Autodesk Inventor part; units mm, degrees
ref_plane "YZ Plane" through (0, 0, 0) normal (1, 0, 0) x (0, 1, 0)
ref_plane "XZ Plane" through (0, 0, 0) normal (0, 1, 0) x (-1, 0, 0)
ref_plane "XY Plane" through (0, 0, 0) normal (0, 0, 1) x (1, 0, 0)
sketch "草圖4" plane through (0, 0, 0) normal (0, 0, 1) x (1, 0, 0)
  line L0 (-29.4, 0) -> (29.4, 0)
  line L1 (0, -7) -> (0, 7)
  line L2 (-21, 5) -> (21, 5)
  line L3 (21, 5) -> (21, -5)
  line L4 (21, -5) -> (-21, -5)
  line L5 (-21, -5) -> (-21, 5)
  circle A0 centre (-11, 0) radius 1.65
  circle A1 centre (11, 0) radius 1.65
  point P0 (0, 0)
  dimension "d20" = 42
  dimension "d21" = 10
  dimension "d22" = 3.3
  dimension "d23" = 3.3
  dimension "d24" = 10
  dimension "d25" = 10
extrude "擠出3" add sketch "草圖4" along normal mid plane 23.5 contours L5 L2 L1 L0 A0 | L0 A0 L1 L4 L5 | L1 L0 A1 L3 L4 | L2 L3 L0 A1 L1
sketch "草圖5" plane through (-21, 5, 11.75) normal (0, 1, 0) x (1, 0, 0)
  line L0 (0, 0) -> (0, 23.5)
  line L1 (42, 0) -> (0, 0)
  line L2 (42, 23.5) -> (42, 0)
  line L3 (0, 23.5) -> (42, 23.5)
  circle A0 centre (21, 11.75) radius 8.5
  circle A1 centre (4.125, 19.25) radius 1.65
  circle A2 centre (4.125, 6.25) radius 1.65
  line L4 (42, 23.5) -> (0, 23.5)
  line L5 (21, 23.5) -> (21, 25.0136)
  circle A3 centre (37.875, 19.25) radius 1.65
  circle A4 centre (37.875, 6.25) radius 1.65
  circle A5 centre (4.125, 19.25) radius 3
  circle A6 centre (4.125, 6.25) radius 3
  circle A7 centre (37.875, 19.25) radius 3
  circle A8 centre (37.875, 6.25) radius 3
  dimension "d28" = 17
  dimension "d31" = 3.3
  dimension "d32" = 3.3
  dimension "d33" = 4.125
  dimension "d34" = 4.25
  dimension "d35" = 6.25
  dimension "d36" = 4.125
  dimension "d37" = 6
  dimension "d38" = 6
extrude "擠出4" cut sketch "草圖5" against normal up to surface (10 mm away) contours A0 | A1 | A2 | A3 | A4
extrude "擠出5" cut sketch "草圖5" against normal blind 4 contours A5 | A6 | A7 | A8
sketch "草圖7" plane through (0, 0, -11.75) normal (0, 0, -1) x (-1, 0, 0)
  circle A0 centre (11, 0) radius 2.75
  circle A1 centre (-11, 0) radius 2.75
  arc A2 (5, -4) -> (-5, -4) centre (0, -12.6603) ccw
  line L0 (18.5, -4) -> (5, -4)
  line L1 (18.5, -4) -> (18.5, 4)
  line L2 (18.5, 4) -> (-18.5, 4)
  line L3 (-18.5, 4) -> (-18.5, -4)
  line L4 (-5, -4) -> (-18.5, -4)
  line L5 (21, -5) -> (21, 5)
  line L6 (21, 5) -> (-21, 5)
  line L7 (-21, 5) -> (-21, -5)
  line L8 (-21, -5) -> (21, -5)
  circle A3 centre (-11, 0) radius 1.65
  circle A4 centre (11, 0) radius 1.65
  arc A5 (4.7245, -5) -> (-4.7245, -5) centre (0, -12.6603) ccw
  line L9 (4.7245, -5) -> (19.5, -5)
  line L10 (19.5, -5) -> (19.5, 5)
  line L11 (19.5, 5) -> (-19.5, 5)
  line L12 (-19.5, 5) -> (-19.5, -5)
  line L13 (-19.5, -5) -> (-4.7245, -5)
  point P0 (0, 0)
  point P1 (-5, -4)
  point P2 (5, -4)
  point P3 (-4.7245, -5)
extrude "擠出7" cut sketch "草圖7" against normal blind 8.65 contours L8 A5
sketch "草圖8" plane through (-21, 5, 11.75) normal (0, 1, 0) x (1, 0, 0)
  circle A0 centre (37.875, 6.25) radius 3
  circle A1 centre (4.125, 6.25) radius 3
  circle A2 centre (21, 11.75) radius 8.5
  line L0 (0, 0) -> (0, 23.5)
  line L1 (42, 0) -> (0, 0)
  line L2 (42, 23.5) -> (42, 0)
  circle A3 centre (21, 11.75) radius 11.5
  line L3 (0, 23.5) -> (42, 23.5)
  dimension "d45" = 23
extrude "擠出8" cut sketch "草圖8" against normal blind 2.5 contours A0 | A1 | A2 | A3
sketch "草圖10" plane through (-21, 5, 11.75) normal (0, 1, 0) x (1, 0, 0)
  circle A0 centre (26.5805, -1.1666) radius 1.5
  circle A1 centre (26.5805, -1.1666) radius 2.75
  point P0 (21, 11.75)
  dimension "d55" = 5.5
extrude "擠出10" cut sketch "草圖10" against normal up to surface (10 mm away) contours A0 | A1
sketch "草圖11" plane through (-21, 5, -11.75) normal (0, 1, 0) x (1, 0, 0)
  circle A0 centre (15.3833, -24.75) radius 1.5
  circle A1 centre (15.3833, -24.75) radius 2.75
  point P0 (21, -11.75)
  dimension "d58" = 5.5
extrude "擠出11" cut sketch "草圖11" against normal up to surface (10 mm away) contours A0 | A1
sketch "草圖12" plane through (-21, 5, -11.75) normal (0, 1, 0) x (1, 0, 0)
  arc A0 (15.8732, -22.044) -> (12.9338, -23.5) centre (15.3833, -24.75) ccw
  arc A1 (26.3579, -21.9256) -> (15.8732, -22.044) centre (21, -11.75) ccw
  arc A2 (29.0708, -23.5) -> (26.3579, -21.9256) centre (26.5805, -24.6666) ccw
  line L0 (42, -23.5) -> (29.0708, -23.5)
  line L1 (42, 0) -> (42, -23.5)
  line L2 (0, 0) -> (42, 0)
  line L3 (0, -23.5) -> (0, 0)
  line L4 (12.9338, -23.5) -> (0, -23.5)
  circle A3 centre (37.875, -17.25) radius 3
  circle A4 centre (4.125, -17.25) radius 3
  circle A5 centre (37.875, -4.25) radius 3
  circle A6 centre (4.125, -4.25) radius 3
  line L5 (42, -23.5) -> (29.0708, -23.5)
  line L6 (29.7708, -23.5) -> (12.2338, -23.5)
  line L7 (12.2338, -23.5) -> (12.2338, -21.2337)
  line L8 (12.2338, -21.2337) -> (29.7708, -21.2337)
  line L9 (29.7708, -21.2337) -> (29.7708, -23.5)
  line L10 (29.7708, -23.5) -> (27.5045, -21.2337)
  line L11 (29.7708, -23.5) -> (32.9758, -23.5) construction
  line L12 (12.2338, -23.5) -> (14.5001, -21.2337)
  line L13 (12.2338, -23.5) -> (15.4388, -23.5) construction
  arc A7 (26.3579, -21.9256) -> (15.8732, -22.044) centre (21, -11.75) ccw
  point P0 (12.9338, -23.5)
  dimension "d62" = 0.7
  dimension "d63" = 0.7
  dimension "d64" = 135
  dimension "d65" = 45
extrude "擠出12" cut sketch "草圖12" against normal up to surface (10 mm away) contours A1 L8 A2 L6 A0 | A0 L4 L12 A1 | A2 A1 L10 L0
properties part number "y_motor_lock_top2_3D 列印"
Could you check a few things on this model? Use its own coordinates, in mm. A direction names the side the tool comes from. Coordinates: 2 decimals unless noted, no trailing zeros. Loops run counter-clockwise (first coordinate to the right, second up) from the corner with the lowest first, then second, coordinate; pieces in that order, holes last.
1. For faces 4 (the face through (-0.07, -3.66, -9.96)), 5 (the face through (7.65, 0.07, 10.63)), 6 (the face through (18, 1, -6)), which set-ups out of +Z, -Z, +X, -X, +Y, -Y let a thin tool reach every point of the face, with its end or its side?
2. Imagine slicing it at A-A (z = 0). Please give me the cut outline in (x, y), and give its area (3 significant figures).
3. Imagine slicing it at C-C (y = -3.25). Give the number of separate pieces and of enclosed holes in the cut face, and give its area (3 significant figures).
4. I need wall thicknesses on L1, parallel to X at y = 3.65, z = 0; L2, parallel to X at y = 2.3, z = 5.5 (3 decimals); L3, parallel to X at y = 2.95, z = 5.5 (1 decimal). Which ranges of each line are inside material? Lowest first, please.
5. For P1, Ø4, axis at x = -0.5, y = 0, coming from the +Z side; P2, Ø3, axis at x = 17.5, z = 6.5, coming from the +Y side, each with a flat end and sliding along its axis, tell me the tip position at first contact or that it passes through.
6. Imagine slicing it at B-B (x = 0). Please give me the cut outline in (y, z).
7. We'd pull the mould along Y, two halves only. Please class faces 1 (the face through (-1, 2.5, -9)), 2 (the face through (0, 0, -11.75)), 3 (the face through (-9.476, 0.632, -0.165)): released by +Y, released by -Y, zero draft, split by the parting line, or undercut.
Computed values:
1. face 4: -Z, -Y
1. face 5: +Z, +Y, -Y
1. face 6: +Y
2. outline: (-21, -5) - (-8.5, -5) - (-8.5, 2.5) - (-11.5, 2.5) - (-11.5, 5) - (-21, 5) - close; (8.5, -5) - (21, -5) - (21, 5) - (11.5, 5) - (11.5, 2.5) - (8.5, 2.5) - close; hole circle Ø3.3 at (-11, 0); hole circle Ø3.3 at (11, 0)
2. area: 218 mm2
3. separate pieces: 1
3. enclosed holes: 5
3. area: 691 mm2
4. L1: x = -21 to -11.5, 11.5 to 21
4. L2: x = -21 to -19.875, -13.875 to -6.481, 6.481 to 13.875, 19.875 to 21
4. L3: x = -21 to -19.9, -13.9 to -10.1, 10.1 to 13.9, 19.9 to 21
5. P1: stops at z = 9.48
5. P2: stops at y = 1
6. outline: (-5, 8.5) - (2.5, 8.5) - (2.5, 9.48) - (-5, 9.48) - close; (-3.66, -11.75) - (5, -11.75) - (5, -11.5) - (2.5, -11.5) - (2.5, -8.5) - (-3.66, -8.5) - close
7. face 1: released by +Y
7. face 2: zero draft
7. face 3: undercut
